Here's the drawing with two shaded views (mm, measured from the low corner). I have some questions. A direction names the side the tool comes from. Coordinates: 2 decimals unless noted, no trailing zeros. Order: outer loops, then holes, each group sorted by start corner. A loop starts at its lowest first (then second) coordinate and runs counter-clockwise, first axis right, second up. Notation, with made-up numbers: M -17.75,15.25 L 18.25,15.25 A8 ccw 18.25,22.25 Z; hole C 24,-23 d9. An arc over 180 degrees is marked long. Put each result on its own line as item: value. Start each with the question number.
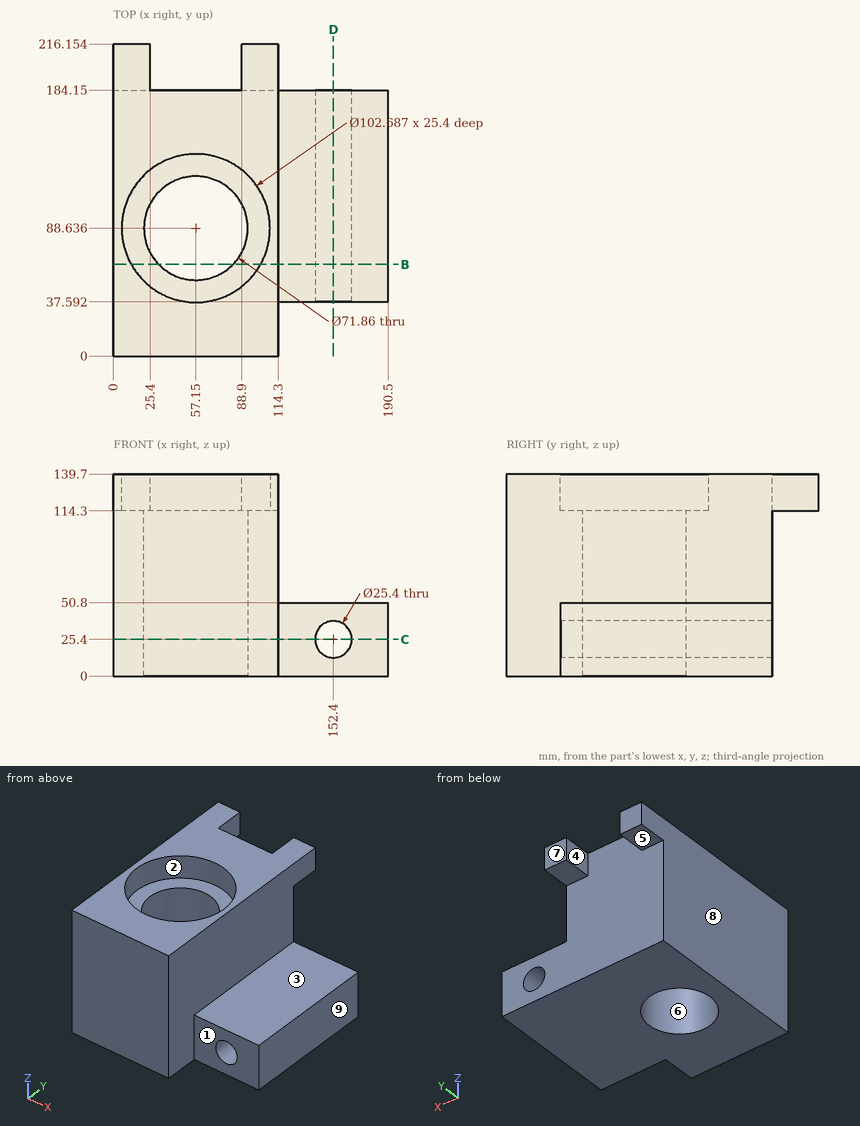
Item 1: If we section it at D-D on x = 152.4: Write out the boundary of the cut face in (y, z), then the cut area to 3 significant figures.
Item 2: For pin 1 Ø4 at (x, z) = (84, 71) entering from +Y; pin 2 Ø7.5 at (y, z) = (204, 124.5) entering from +X; pin 3 Ø12 at (x, y) = (163.5, 108.5) entering from +Z, each with a flat end and sliding along its axis, tell me the tip position at first contact or that it passes through.
Item 3: I need wall thicknesses on probe 1 along Y at (x, z) = (57.15, 128.5); probe 2 along X at (y, z) = (85, 31) (1 decimal); probe 3 along Z at (x, y) = (39, 121). Which ranges of each line are inside material? Lowest first, please.
Item 4: If we mould it in two halves opening along X, with no side actions, what happens to the marked faces 6, 7, 8 and 9? For each: released by +X, released by -X, zero draft, split by the parting line, or undercut.
Item 5: If we section it at B-B on y = 63.5: Write out the boundary of the cut face in (x, z) (1 decimal).
Item 6: For the marked faces 1, 2, 3, 4 and 5, which set-ups out of +Z, -Z, +X, -X, +Y, -Y let a thin tool reach every point of the face, with its end or its side?
Item 7: If we section it at C-C on z = 25.4: State how many separate pieces and enclosed holes the cut face has, then the cut area to 3 significant figures.
Geometry check:
1. outline: M 37.59,0 L 184.15,0 L 184.15,12.7 L 37.59,12.7 Z; M 37.59,38.1 L 184.15,38.1 L 184.15,50.8 L 37.59,50.8 Z
1. area: 3,720 mm²
2. pin 1: stops at y = 184.15
2. pin 2: stops at x = 114.3
2. pin 3: stops at z = 50.8
3. probe 1: y = 0 to 37.29, 139.98 to 184.15
3. probe 2: x = 0 to 21.4, 92.9 to 141, 163.8 to 190.5
3. probe 3: z = 0 to 114.3
4. face 6: undercut
4. face 7: zero draft
4. face 8: released by -X
4. face 9: released by +X
5. outline: M 0,0 L 31.5,0 L 31.5,114.3 L 12.4,114.3 L 12.4,139.7 L 0,139.7 Z; M 82.8,0 L 190.5,0 L 190.5,50.8 L 114.3,50.8 L 114.3,139.7 L 101.9,139.7 L 101.9,114.3 L 82.8,114.3 Z; hole C 152.4,25.4 d25.4
6. face 1: +Z, -Z, +X, -Y
6. face 2: +Z
6. face 3: +Z, +X, +Y, -Y
6. face 4: +Z, -Z, +Y
6. face 5: -Z, +X, -X, +Y
7. separate pieces: 2
7. enclosed holes: 1
7. area: 24,400 mm²
